Work out the finished part from the listing and answer in its coordinate system (mm). A direction names the side the tool comes from. Coordinates: 2 decimals unless noted, no trailing zeros. Order: outer loops, then holes, each group sorted by start corner. A loop starts at its lowest first (then second) coordinate and runs counter-clockwise, first axis right, second up.
```python
from build123d import *

# Parameters (mm, degrees)
SKETCH1_R           = 5
SKETCH1_R_2         = 2.5
BOSS_EXTRUDE1_DEPTH = 5
FILLET1_R           = 5


with BuildPart() as part:
    # Sketch1 → Boss-Extrude1 (new body)
    # profile 1 of 3: a face of its own
    with BuildSketch(Plane.XY):
        with BuildLine():
            Line((-7.5, 3.349364905), (-7.5, 35))
            ThreePointArc((-7.5, 35), (-12.5, 30), (-17.5, 35))
            Line((-17.5, 35), (-17.5, -4.323904974))
            Line((-17.5, -4.323904974), (7.5, -11.022634785))
            Line((7.5, -11.022634785), (7.5, -35))
            ThreePointArc((7.5, -35), (12.5, -30), (17.5, -35))
            Line((17.5, -35), (17.5, -3.349364905))
            Line((17.5, -3.349364905), (-7.5, 3.349364905))
        make_face()
    # profile 2 of 3: a face of its own
    with BuildSketch(Plane.XY):
        with Locations((-12.5, 35)):
            Circle(SKETCH1_R)
        with Locations((-12.5, 35)):
            Circle(SKETCH1_R_2, mode=Mode.SUBTRACT)
    # profile 3 of 3: a face of its own
    with BuildSketch(Plane.XY):
        with Locations((12.5, -35)):
            Circle(SKETCH1_R)
        with Locations((12.5, -35)):
            Circle(SKETCH1_R_2, mode=Mode.SUBTRACT)
    extrude(amount=BOSS_EXTRUDE1_DEPTH)

    # Fillet1
    fillet1_edges = [part.edges().sort_by_distance(p)[0] for p in [
        (-7.5, 3.349364905, 2.5),
        (17.5, -3.349364905, 2.5),
        (7.5, -11.022634785, 2.5),
        (-17.5, -4.323904974, 2.5),
    ]]
    fillet(fillet1_edges, radius=FILLET1_R)


solid = part.part
```
1. For faces 1 (the flat face through (7.5, -25, 2)), 2 (the flat face through (-7.5, 21, 2)), 3 (the flat face through (0, -3, 0)), determine the directions among +Z, -Z, +X, -X, +Y, -Y from which every point of the face is accessible in a straight line to the end or side of a thin tool.
2. Flat-ended cylindrical pins translate along their axes: pin 1 (1 mm diameter, centred on x = -14, z = 3.5, fed in from -Y); pin 2 (2.5 mm diameter, centred on y = -25.5, z = 2.5, fed in from -X); pin 3 (3 mm diameter, centred on y = -6, z = 4.5, fed in from -X); pin 4 (12 mm diameter, centred on x = 12.5, y = -6.5, fed in from -Z). Find the tip coordinate at first contact, or state that the pin passes through.
3. The part is cut by section C-C (y = -24.5). Determine the outline of the cut face in (x, z).
4. Consider probe 1 along X at (y, z) = (-30, 4.35); probe 2 along X at (y, z) = (10, 1.85); probe 3 along Y at (x, z) = (12.5, 2). Determine where each line is inside the solid, lowest interval first.
5. The part is cut by section B-B (x = 12.5). Determine the outline of the cut face in (y, z), plus the area to 3 significant figures.
6. The mould has two halves that part along X. Classify faces 4 (the cylindrical face through (-12.4, 40, 2.5)), 5 (the cylindrical face through (11, -33, 2)), 6 (the flat face through (-17.5, 18, 2)): released by +X, released by -X, zero draft, split by the parting line, or undercut.
7. The part is cut by section D-D (x = -12.5). Determine the outline of the cut face in (y, z), plus the area to 3 significant figures.
8. The part is cut by section A-A (z = 3.45). Determine the outline of the cut face in (x, y).
Worked out:
1. face 1: +Z, -Z, -X, -Y
1. face 2: +Z, -Z, +X, +Y
1. face 3: -Z, +X, -X, +Y, -Y
2. pin 1: stops at y = -5.4
2. pin 2: stops at x = 7.5
2. pin 3: stops at x = -15.48
2. pin 4: stops at z = 0
3. outline: (7.5, 0) - (17.5, 0) - (17.5, 5) - (7.5, 5) - close
4. probe 1: x = 7.5 to 17.5
4. probe 2: x = -17.5 to -7.5
4. probe 3: y = -40 to -37.5, -32.5 to -2.01
5. outline: (-40, 0) - (-37.5, 0) - (-37.5, 5) - (-40, 5) - close; (-32.5, 0) - (-2.01, 0) - (-2.01, 5) - (-32.5, 5) - close
5. area: 165 mm2
6. face 4: split by the parting line
6. face 5: undercut
6. face 6: released by -X
7. outline: (-5.66, 0) - (32.5, 0) - (32.5, 5) - (-5.66, 5) - close; (37.5, 0) - (40, 0) - (40, 5) - (37.5, 5) - close
7. area: 203 mm2
8. outline: (-17.5, -0.49) arc R5 ccw to (-13.79, -5.32) - (3.79, -10.03) arc R5 cw to (7.5, -14.86) - (7.5, -35) arc R5 ccw to (17.5, -35) - (17.5, -7.19) arc R5 ccw to (13.79, -2.36) - (-3.79, 2.36) arc R5 cw to (-7.5, 7.19) - (-7.5, 35) arc R5 ccw to (-17.5, 35) - close; hole circle Ø5 at (-12.5, 35); hole circle Ø5 at (12.5, -35)
